Autodesk Fusion 360 part; units mm, degrees
sketch "Sketch1" plane through (0, 0, 0) normal (0, 0, 1) x (1, 0, 0)
  circle A0 centre (0, 0) radius 2.35
  circle A1 centre (0, 0) radius 3.5
  dimension "d1" = 4.7
  dimension "d4" = 7
extrude "Extrude1" add sketch "Sketch1" along normal blind 8 contours A0
extrude "Extrude2" add sketch "Sketch1" against normal blind 13 contours A0 | A1
ref_plane "WorkPlane1" through (0, 0, -15) normal (0, 0, 1) x (1, 0, 0)
sketch "Sketch2" plane through (0, 0, -15) normal (0, 0, 1) x (1, 0, 0)
  circle A0 centre (0, 0) radius 1.9
  dimension "d8" = 3.8
extrude "Extrude3" cut sketch "Sketch2" along normal blind 8
fillet "Fillet1" radius 1 1 edges at (-2.191, -0.8498, 8)
Geometry: final body of the model. Coordinates: model frame, mm. A direction names the side the tool comes from. Coordinates: 2 decimals unless noted, no trailing zeros. Order: outer loops, then holes, each group sorted by start corner. A loop starts at its lowest first (then second) coordinate and runs counter-clockwise, first axis right, second up. Notation, with made-up numbers: (63.5, -6.5) -> (121.5, -6.5) arc R5 cw to (121.5, 2.5) -> close; hole circle Ø5 at (66, 42.5). An arc over 180 degrees is marked (long way). Answer in a Markdown table with one row per item.
Item 1: Section A-A on x = 0. Output: boundary loops of the cut face in (y, z).
Return value:
| item | result |
|---|---|
| outline | (-3.5, -13) -> (-1.9, -13) -> (-1.9, -7) -> (1.9, -7) -> (1.9, -13) -> (3.5, -13) -> (3.5, 0) -> (2.35, 0) -> (2.35, 7) arc R1 ccw to (1.35, 8) -> (-1.35, 8) arc R1 ccw to (-2.35, 7) -> (-2.35, 0) -> (-3.5, 0) -> close |
Item 2: Section D-D on z = -3.25. Output: boundary loops of the cut face in (x, y).
Return value:
| item | result |
|---|---|
| outline | circle Ø7 at (0, 0) |
Item 3: Section C-C on z = -11. Output: boundary loops of the cut face in (x, y).
Return value:
| item | result |
|---|---|
| outline | circle Ø7 at (0, 0); hole circle Ø3.8 at (0, 0) |
Item 4: Draft query along X for faces 1 (the flat face through (2, -2, -13)), 2 (the cylindrical face through (-1.9, -0.08, -10.04)), 3 (the cylindrical face through (3.233, -1.341, -6.409)). Return one class per face: released by +X, released by -X, zero draft, split by the parting line, or undercut.
Return value:
| item | result |
|---|---|
| face 1 | zero draft |
| face 2 | undercut |
| face 3 | split by the parting line |
Item 5: Ray query, L1, parallel to Y at x = 0, z = -9.35; L2, parallel to Z at x = 0, y = -1.25; L3, parallel to Z at x = -2.5, y = -2. Return the intervals inside material, ascending.
Return value:
| item | result |
|---|---|
| L1 | y = -3.5 to -1.9, 1.9 to 3.5 |
| L2 | z = -7 to 8 |
| L3 | z = -13 to 0 |
Item 6: Access query for faces 4 (the flat face through (0, 0, 8)), 5 (the flat face through (0, 0, -7)), 6 (the cylindrical face through (-0.509, 2.294, 3.451)). Directions: +Z, -Z, +X, -X, +Y, -Y. A direction counts if a zero-diameter tool reaches every point of the face in a straight line with its end or side. Return the directions, or none.
Return value:
| item | result |
|---|---|
| face 4 | +Z, +X, -X, +Y, -Y |
| face 5 | -Z |
| face 6 | +Z |
Item 7: Contact query for flat-ended pins moving along their axis: P1, Ø3, axis at y = -2.5, z = -6.5, coming from the +X side; P2, Ø2, axis at x = 2.5, y = 2.5, coming from the +Z side; P3, Ø1, axis at x = -2, z = -5, coming from the -Y side. Output: stop coordinate, or through.
Return value:
| item | result |
|---|---|
| P1 | stops at x = 3.35 |
| P2 | stops at z = 0 |
| P3 | stops at y = -3.16 |
